Build history of the part. All positions in model axes, mm. Face numbers are marked on the shaded views. Round coordinates to 2 decimals unless told otherwise and drop trailing zeros. Write each loop counter-clockwise with the first axis right and the second up, starting at its lowest first coordinate (ties: lowest second). Pieces come first, ordered by that corner, then holes. Notation, with made-up numbers: (23, 27) - (53, 27) arc R15 ccw to (53, 32) - close; hole circle Ø2 at (-20.5, 0.25). An arc over 180 degrees is marked (long way). One line per question, with ' | ' between items.
from build123d import *

# Parameters (mm, degrees)
F0_W     = 115
F0_H     = 40
F0_W_2   = 105
F0_H_2   = 30
F1_DEPTH = 5
F2_DEPTH = 22
F3_R     = 2
F5_DEPTH = 105


with BuildPart() as f1:
    # F0 (on Top) → F1 (new body)
    with BuildSketch(Plane.XY):
        Rectangle(F0_W, F0_H)
        Rectangle(F0_W_2, F0_H_2, mode=Mode.SUBTRACT)
        Rectangle(F0_W_2, F0_H_2)
    extrude(amount=-F1_DEPTH)

    # F0 (on Top) → F2 (join)
    with BuildSketch(Plane.XY):
        Rectangle(F0_W, F0_H)
        Rectangle(F0_W_2, F0_H_2, mode=Mode.SUBTRACT)
    extrude(amount=F2_DEPTH)

    # F3
    f3_edges = [f1.edges().sort_by_distance(p)[0] for p in [
        (0, 20, 22),
        (-57.5, 0, 22),
        (0, -20, 22),
        (57.5, 0, 22),
    ]]
    fillet(f3_edges, radius=F3_R)

    # F4 (on face) → F5 (join, through all)
    with BuildSketch(Plane(origin=(52.5, 0, 0), x_dir=(0, -1, 0), z_dir=(-1, 0, 0))):
        with BuildLine():
            Line((-15, 1.9643241272), (-15, 0))
            Line((-15, 0), (15, 0))
            Line((15, 0), (15, 1.9643241272))
            add(Edge.make_bspline(
                [(15, 1.9643241272), (9, 1), (0, 6), (-9, 1), (-15, 1.9643241272)],
                knots=[0, 0, 0, 0, 0.5, 1, 1, 1, 1], degree=3))
        make_face()
    extrude(amount=F5_DEPTH)


solid = f1.part
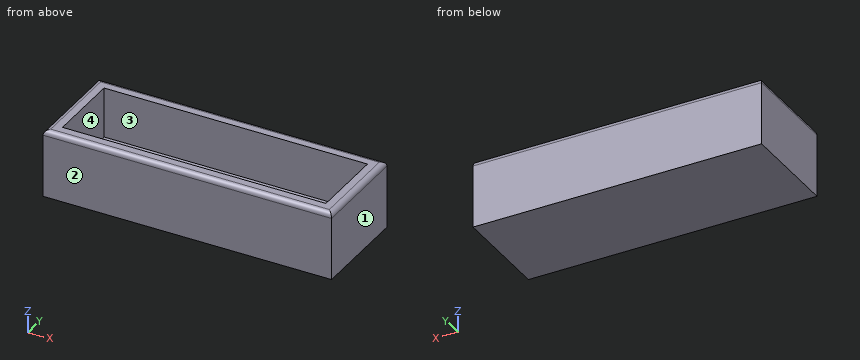
Q1. Pull direction Y, two halves, no side cores. Call the marked faces 1, 2, 3 and 4: +Y half, -Y half, draft (parallel to the pull), parting line (faces both ways), or undercut.
Found:
face 1: draft | face 2: -Y half | face 3: undercut | face 4: undercut
Q2. Drill centre lines: L1, parallel to Y at x = -16.5, z = 7.75; L2, parallel to X at y = -14.5, z = 17.5; L3, parallel to Z at x = 47, y = 0. Where is each one in solid material? Low to high. Write a range as from..to.
Found:
L1: -20..-15, 15..20 | L2: -57.5..-52.5, 52.5..57.5 | L3: -5..3.5
Q3. Saw through at A-A, the plane z = 10. List the corners of the cut face in (x, y).
Found:
outline: (-57.5, -20) - (57.5, -20) - (57.5, 20) - (-57.5, 20) - close; hole (-52.5, -15) - (52.5, -15) - (52.5, 15) - (-52.5, 15) - close
